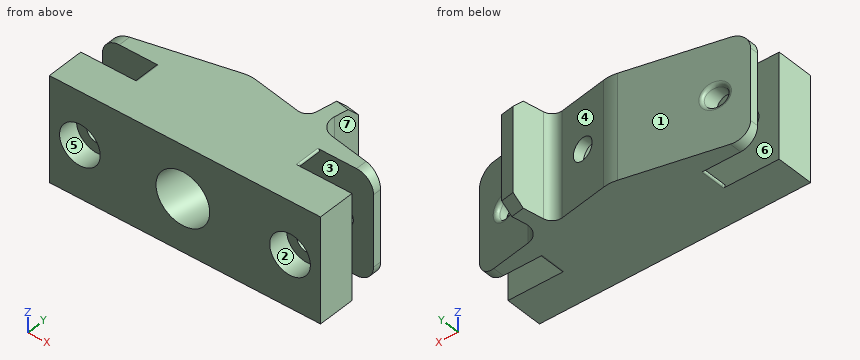
from build123d import *

# Parameters (mm, degrees)
SKETCH1_W           = 80
SKETCH1_H           = 31
SKETCH1_R           = 6
BOSS_EXTRUDE1_DEPTH = 6
SKETCH2_W           = 80
SKETCH2_H           = 31
SKETCH2_R           = 3.05
BOSS_EXTRUDE2_DEPTH = 5.9
BOSS_EXTRUDE3_DEPTH = 6.8
FILLET1_R           = 0.5
SKETCH4_W           = 80
SKETCH4_H           = 31
SKETCH4_R           = 3.05
BOSS_EXTRUDE4_DEPTH = 2.5
BOSS_EXTRUDE5_DEPTH = 31
SKETCH6_R           = 3.3
CUT_EXTRUDE1_DEPTH  = 48
SKETCH7_R           = 7.8
CUT_EXTRUDE2_DEPTH  = 47
BOSS_EXTRUDE6_DEPTH = 31
FILLET2_R           = 3
FILLET3_R           = 5
CHAMFER1_SIZE       = 3
FILLET4_R           = 5
FILLET5_R           = 10
SKETCH9_R           = 3.05
CUT_EXTRUDE3_DEPTH  = 32.549910473
FILLET6_R           = 1
CUT_EXTRUDE4_DEPTH  = 0.8


with BuildPart() as part:
    # Sketch1 → Boss-Extrude1 (new body)
    with BuildSketch(Plane(origin=(0, 0, 0), x_dir=(1, 0, 0), z_dir=(0, 1, 0))):
        Rectangle(SKETCH1_W, SKETCH1_H)
        with Locations((-31, 0)):
            Circle(SKETCH1_R, mode=Mode.SUBTRACT)
        with Locations((31, 0)):
            Circle(SKETCH1_R, mode=Mode.SUBTRACT)
    extrude(amount=BOSS_EXTRUDE1_DEPTH)

    # Sketch2 → Boss-Extrude2 (add)
    with BuildSketch(Plane(origin=(0, 6, 0), x_dir=(1, 0, 0), z_dir=(0, 1, 0))):
        Rectangle(SKETCH2_W, SKETCH2_H)
        with Locations((-31, 0)):
            Circle(SKETCH2_R, mode=Mode.SUBTRACT)
        with Locations((31, 0)):
            Circle(SKETCH2_R, mode=Mode.SUBTRACT)
    extrude(amount=BOSS_EXTRUDE2_DEPTH)

    # Sketch3 → Boss-Extrude3 (add)
    with BuildSketch(Plane(origin=(0, 11.9, 0), x_dir=(1, 0, 0), z_dir=(0, 1, 0))):
        with BuildLine():
            ThreePointArc((26.120194676, -15.5), (14.75, 0), (26.120194676, 15.5))
            Line((26.120194676, 15.5), (-26.120194676, 15.5))
            ThreePointArc((-26.120194676, 15.5), (-17.897341176, 9.611598813), (-14.75, 0))
            ThreePointArc((-14.75, 0), (-17.897341176, -9.611598813), (-26.120194676, -15.5))
            Line((-26.120194676, -15.5), (26.120194676, -15.5))
        make_face()
    extrude(amount=BOSS_EXTRUDE3_DEPTH)

    # Fillet1
    fillet1_edges = [part.edges().sort_by_distance(p)[0] for p in [
        (26.120194676, 15.3, 15.5),
        (26.120194676, 15.3, -15.5),
        (-26.120194676, 15.3, -15.5),
        (-26.120194676, 15.3, 15.5),
    ]]
    fillet(fillet1_edges, radius=FILLET1_R)

    # Sketch4 → Boss-Extrude4 (add)
    with BuildSketch(Plane(origin=(0, 18.7, 0), x_dir=(1, 0, 0), z_dir=(0, 1, 0))):
        Rectangle(SKETCH4_W, SKETCH4_H)
        with Locations((-31, 0)):
            Circle(SKETCH4_R, mode=Mode.SUBTRACT)
        with Locations((31, 0)):
            Circle(SKETCH4_R, mode=Mode.SUBTRACT)
    extrude(amount=BOSS_EXTRUDE4_DEPTH)

    # Sketch5 → Boss-Extrude5 (add)
    with BuildSketch(Plane.XY.offset(15.5)):
        Polygon((40, 21.2), (-5, 29.134714132), (-40, 21.2), align=None)
    extrude(amount=-BOSS_EXTRUDE5_DEPTH)

    # Sketch6 → Cut-Extrude1 (cut)
    with BuildSketch(Plane(origin=(4.831561104, 27.401144647, 0), x_dir=(0.984807753, -0.173648178, 0), z_dir=(0.173648178, 0.984807753, 0))):
        with Locations((-0.60768988, 0)):
            Circle(SKETCH6_R)
    extrude(amount=-CUT_EXTRUDE1_DEPTH, mode=Mode.SUBTRACT)

    # Sketch7 → Cut-Extrude2 (cut)
    with BuildSketch(Plane(origin=(-3.85084778, -21.839243004, 0), x_dir=(0.984807753, -0.173648178, 0), z_dir=(0.173648178, 0.984807753, 0))):
        with Locations((-0.60768988, 0)):
            Circle(SKETCH7_R)
    extrude(amount=CUT_EXTRUDE2_DEPTH, mode=Mode.SUBTRACT)

    # Sketch8 → Boss-Extrude6 (add)
    with BuildSketch(Plane.XY.offset(15.5)):
        Polygon((14.296517646, 25.732217437), (16.380295778, 37.549910473), (20.31952679, 36.855317763), (18.235748658, 25.037624726), align=None)
    extrude(amount=-BOSS_EXTRUDE6_DEPTH)

    # Fillet2
    fillet2_edges = [part.edges().sort_by_distance(p)[0] for p in [
        (14.296517646, 25.732217437, 0),
    ]]
    fillet(fillet2_edges, radius=FILLET2_R)

    # Fillet3
    fillet3_edges = [part.edges().sort_by_distance(p)[0] for p in [
        (18.235748658, 25.037624726, 0),
    ]]
    fillet(fillet3_edges, radius=FILLET3_R)

    # Chamfer1
    chamfer1_edges = [part.edges().sort_by_distance(p)[0] for p in [
        (18.349911284, 37.202614118, 15.5),
        (18.349911284, 37.202614118, -15.5),
    ]]
    chamfer(chamfer1_edges, length=CHAMFER1_SIZE)

    # Fillet4
    fillet4_edges = [part.edges().sort_by_distance(p)[0] for p in [
        (-40, 19.95, -15.5),
        (-40, 19.95, 15.5),
        (40, 19.95, 15.5),
        (40, 19.95, -15.5),
    ]]
    fillet(fillet4_edges, radius=FILLET4_R)

    # Fillet5
    fillet5_edges = [part.edges().sort_by_distance(p)[0] for p in [
        (-5, 29.134714132, 0),
    ]]
    fillet(fillet5_edges, radius=FILLET5_R)

    # Sketch9 → Cut-Extrude3 (cut, through all)
    with BuildSketch(Plane.XZ.offset(-6)):
        with Locations((-31, 0)):
            Circle(SKETCH9_R)
        with Locations((31, 0)):
            Circle(SKETCH9_R)
    extrude(amount=-CUT_EXTRUDE3_DEPTH, mode=Mode.SUBTRACT)

    # Fillet6
    fillet6_edges = [part.edges().sort_by_distance(p)[0] for p in [
        (27.95, 23.324740118, 2.44e-07),
        (-34.05, 22.548901402, 8.61e-07),
    ]]
    fillet(fillet6_edges, radius=FILLET6_R)

    # Sketch10 → Cut-Extrude4 (cut)
    with BuildSketch(Plane(origin=(0, 11.9, 0), x_dir=(1, 0, 0), z_dir=(0, 1, 0))):
        with BuildLine():
            Line((40, 15.5), (23.545974242, 15.5))
            ThreePointArc((23.545974242, 15.5), (24.032739379, 15.114279051), (23.768482474, 14.552238806))
            ThreePointArc((23.768482474, 14.552238806), (14.75, 0), (23.768482474, -14.552238806))
            ThreePointArc((23.768482474, -14.552238806), (24.032739379, -15.114279051), (23.545974242, -15.5))
            Line((23.545974242, -15.5), (40, -15.5))
            Line((40, -15.5), (40, 15.5))
        make_face()
        with BuildLine():
            Line((-40, -15.5), (-23.545974242, -15.5))
            ThreePointArc((-23.545974242, -15.5), (-24.032739379, -15.114279051), (-23.768482474, -14.552238806))
            ThreePointArc((-23.768482474, -14.552238806), (-14.75, 0), (-23.768482474, 14.552238806))
            ThreePointArc((-23.768482474, 14.552238806), (-24.032739379, 15.114279051), (-23.545974242, 15.5))
            Line((-23.545974242, 15.5), (-40, 15.5))
            Line((-40, 15.5), (-40, -15.5))
        make_face()
    extrude(amount=-CUT_EXTRUDE4_DEPTH, mode=Mode.SUBTRACT)


solid = part.part
Could you check a few things on this model? Use its own coordinates, in mm. Face numbers are marked on the shaded views. A direction names the side the tool comes from. Coordinates: 2 decimals unless noted, no trailing zeros. Answer in a Markdown table with one row per item. Add a question column.
(1) If we section it at A-A, the plane x = 31: State how many separate pieces and enclosed holes the cut face has, then the cut area to 3 significant figures.
(2) Will these pins go through, and if not, where does the flat tip stop? pin 1 (9.5 mm diameter, centred on x = 29.5, z = 0, fed in from -Y); pin 2 (12.5 mm diameter, centred on x = -26, z = 0.5, fed in from +Y); pin 3 (11 mm diameter, centred on x = -31, z = 0, fed in from +Y); pin 4 (5 mm diameter, centred on x = 1, z = 3.5, fed in from +Y).
(3) I need wall thicknesses on L1, parallel to Z at x = 31, y = 2.35; L2, parallel to Z at x = -31, y = 7.9; L3, parallel to X at y = 7.2, z = 0. Which ranges of each line are inside material? Lowest first, please.
(4) On a 3-axis mill with a long thin cutter (end or side, diameter ignored), from which of +Z, -Z, +X, -X, +Y, -Y can I reach the whole of each face in a straight line? I mean the marked faces 4, 5, 6 and 7. Say none if no direction works.
(5) If we mould it in two halves opening along X, with no side actions, what happens to the marked faces 1, 2 and 3? For each: released by +X, released by -X, zero draft, split by the parting line, or undercut.
Results are:
| question | item | result |
|---|---|---|
| 1 | separate pieces | 4 |
| 1 | enclosed holes | 0 |
| 1 | area | 342 mm2 |
| 2 | pin 1 | stops at y = 0 |
| 2 | pin 2 | stops at y = 25.79 |
| 2 | pin 3 | stops at y = 24.49 |
| 2 | pin 4 | stops at y = 28.52 |
| 3 | L1 | z = -15.5 to -6, 6 to 15.5 |
| 3 | L2 | z = -15.5 to -3.05, 3.05 to 15.5 |
| 3 | L3 | x = -40 to -34.05, -27.95 to -7.27, 8.57 to 27.95, 34.05 to 40 |
| 4 | face 4 | +Z, -Z, +Y |
| 4 | face 5 | -Y |
| 4 | face 6 | -X |
| 4 | face 7 | +Z, -Z, +X |
| 5 | face 1 | released by -X |
| 5 | face 2 | undercut |
| 5 | face 3 | zero draft |
